Geometry: final body of the model. Coordinates: model frame, mm. A direction names the side the tool comes from. Give positions to 0.01 mm unless a question says otherwise; leave off trailing zeros. Write each loop counter-clockwise with the first axis right and the second up, starting at its lowest first coordinate (ties: lowest second). Pieces come first, ordered by that corner, then holes.
Q1. Draft query along Y for faces 3 (the face through (50, 5, 9)), 4 (the face through (97.167, 57.097, 3.507)), 5 (the face through (98.5, 1.43, 3.51)). Return one class per face: pulls with the +Y half, pulls with the -Y half, needs draft (parallel to the pull), parting line crosses it, or undercut.
Q2. Pin query (flat end, axial travel): pin 1 (3 mm diameter, centred on y = 31, z = 7, fed in from -X); pin 2 (2 mm diameter, centred on x = 38.5, z = 5.5, fed in from -Y); pin 3 (1.5 mm diameter, centred on x = 33, z = 5.5, fed in from +Y). Return the tip coordinate at first contact, or that it passes through.
Q3. Line query: L1, parallel to X at y = 44.5, z = 6.5; L2, parallel to Y at x = 64.5, z = 7.25; L3, parallel to X at y = 55.5, z = 3.25. Output: solid intervals per line, ascending.
Q4. Cut plane B-B on y = 16.5. Return the cut outline in (x, z).
Q5. Reachability of faces 1 (the face through (1.43, 1.5, 3.51)), 2 (the face through (96.95, 30, 5)) from +Z, -Z, +X, -X, +Y, -Y: full face, straight path, thin tool, end or side. Return the list, or none.
Q6. Cut plane A-A on z = 5.5. Return the cut outline in (x, y), plus the area to 3 significant figures.
Q7. Cut plane C-C on x = 35.5. Return the cut outline in (y, z), plus the area to 3 significant figures.
```python
from build123d import *

# Parameters (mm, degrees)
SKETCH_W        = 100
SKETCH_H        = 60
PAD_DEPTH       = 4
FILLET_R        = 5
FILLET001_R     = 3
POCKET001_DEPTH = 1
PAD001_DEPTH    = 5
POCKET_DEPTH    = 6
FILLET002_R     = 1


with BuildPart() as part:
    # Sketch → Pad (new body)
    with BuildSketch(Plane.XY):
        with Locations((50, 30)):
            Rectangle(SKETCH_W, SKETCH_H)
    extrude(amount=PAD_DEPTH)

    # Fillet
    fillet_edges = [part.edges().sort_by_distance(p)[0] for p in [
        (100, 0, 2),
        (0, 0, 2),
        (100, 60, 2),
        (0, 60, 2),
    ]]
    fillet(fillet_edges, radius=FILLET_R)

    # Fillet001
    fillet001_edges = [part.edges().sort_by_distance(p)[0] for p in [
        (50, 60, 0),
    ]]
    fillet(fillet001_edges, radius=FILLET001_R)

    # Sketch008 (on Face6 of Pad) → Pocket001 (cut)
    with BuildSketch(Plane.XY.offset(4)):
        with BuildLine():
            Line((6.05, 1.55), (93.95, 1.55))
            ThreePointArc((93.95, 1.55), (97.131981, 2.868019), (98.45, 6.05))
            Line((98.45, 6.05), (98.45, 53.95))
            ThreePointArc((98.45, 53.95), (97.131981, 57.131981), (93.95, 58.45))
            Line((93.95, 58.45), (6.05, 58.45))
            ThreePointArc((6.05, 58.45), (2.868019, 57.131981), (1.55, 53.95))
            Line((1.55, 53.95), (1.55, 6.05))
            ThreePointArc((1.55, 6.05), (2.868019, 2.868019), (6.05, 1.55))
        make_face()
        with BuildLine():
            Line((6.05, 3.05), (93.95, 3.05))
            ThreePointArc((93.95, 3.05), (96.07132, 3.92868), (96.95, 6.05))
            Line((96.95, 6.05), (96.95, 53.95))
            ThreePointArc((96.95, 53.95), (96.07132, 56.07132), (93.95, 56.95))
            Line((93.95, 56.95), (6.05, 56.95))
            ThreePointArc((6.05, 56.95), (3.92868, 56.07132), (3.05, 53.95))
            Line((3.05, 53.95), (3.05, 6.05))
            ThreePointArc((3.05, 6.05), (3.92868, 3.92868), (6.05, 3.05))
        make_face(mode=Mode.SUBTRACT)
    extrude(amount=-POCKET001_DEPTH, mode=Mode.SUBTRACT)

    # Sketch001 (on Face6 of Pad) → Pad001 (join)
    with BuildSketch(Plane.XY.offset(4)):
        with BuildLine():
            Line((6.05, 3.05), (93.95, 3.05))
            ThreePointArc((93.95, 3.05), (96.07132, 3.92868), (96.95, 6.05))
            Line((96.95, 6.05), (96.95, 53.95))
            ThreePointArc((96.95, 53.95), (96.07132, 56.07132), (93.95, 56.95))
            Line((93.95, 56.95), (6.05, 56.95))
            ThreePointArc((6.05, 56.95), (3.92868, 56.07132), (3.05, 53.95))
            Line((3.05, 53.95), (3.05, 6.05))
            ThreePointArc((3.05, 6.05), (3.92868, 3.92868), (6.05, 3.05))
        make_face()
    extrude(amount=PAD001_DEPTH)

    # Sketch009 (on Face44 of Pad001) → Pocket (cut)
    with BuildSketch(Plane.XY.offset(9)):
        with BuildLine():
            Line((7.5, 5.5), (92.5, 5.5))
            ThreePointArc((92.5, 5.5), (93.914214, 6.085786), (94.5, 7.5))
            Line((94.5, 7.5), (94.5, 52.5))
            ThreePointArc((94.5, 52.5), (93.914214, 53.914214), (92.5, 54.5))
            Line((92.5, 54.5), (7.5, 54.5))
            ThreePointArc((7.5, 54.5), (6.085786, 53.914214), (5.5, 52.5))
            Line((5.5, 52.5), (5.5, 7.5))
            ThreePointArc((5.5, 7.5), (6.085786, 6.085786), (7.5, 5.5))
        make_face()
    extrude(amount=-POCKET_DEPTH, mode=Mode.SUBTRACT)

    # Fillet002
    fillet002_edges = [part.edges().sort_by_distance(p)[0] for p in [
        (50, 3.05, 9),
    ]]
    fillet(fillet002_edges, radius=FILLET002_R)


solid = part.part
```
Data:
1. face 3: needs draft
1. face 4: undercut
1. face 5: pulls with the -Y half
2. pin 1: stops at x = 3.05
2. pin 2: stops at y = 3.05
2. pin 3: stops at y = 56.95
3. L1: x = 3.05 to 5.5, 94.5 to 96.95
3. L2: y = 3.05 to 5.5, 54.5 to 56.95
3. L3: x = 0.03 to 1.83, 3.48 to 96.52, 98.17 to 99.97
4. outline: (0, 3) arc R3 ccw to (3, 0) - (97, 0) arc R3 ccw to (100, 3) - (100, 4) - (98.45, 4) - (98.45, 3) - (96.95, 3) - (96.95, 8) arc R1 ccw to (95.95, 9) - (94.5, 9) - (94.5, 3) - (5.5, 3) - (5.5, 9) - (4.05, 9) arc R1 ccw to (3.05, 8) - (3.05, 3) - (1.55, 3) - (1.55, 4) - (0, 4) - close
5. face 1: +Z, -Z, -X, -Y
5. face 2: +Z
6. outline: (3.05, 6.05) arc R3 ccw to (6.05, 3.05) - (93.95, 3.05) arc R3 ccw to (96.95, 6.05) - (96.95, 53.95) arc R3 ccw to (93.95, 56.95) - (6.05, 56.95) arc R3 ccw to (3.05, 53.95) - close; hole (5.5, 7.5) arc R2 ccw to (7.5, 5.5) - (92.5, 5.5) arc R2 ccw to (94.5, 7.5) - (94.5, 52.5) arc R2 ccw to (92.5, 54.5) - (7.5, 54.5) arc R2 ccw to (5.5, 52.5) - close
6. area: 696 mm2
7. outline: (0, 3) arc R3 ccw to (3, 0) - (57, 0) arc R3 ccw to (60, 3) - (60, 4) - (58.45, 4) - (58.45, 3) - (56.95, 3) - (56.95, 8) arc R1 ccw to (55.95, 9) - (54.5, 9) - (54.5, 3) - (5.5, 3) - (5.5, 9) - (4.05, 9) arc R1 ccw to (3.05, 8) - (3.05, 3) - (1.55, 3) - (1.55, 4) - (0, 4) - close
7. area: 208 mm2
